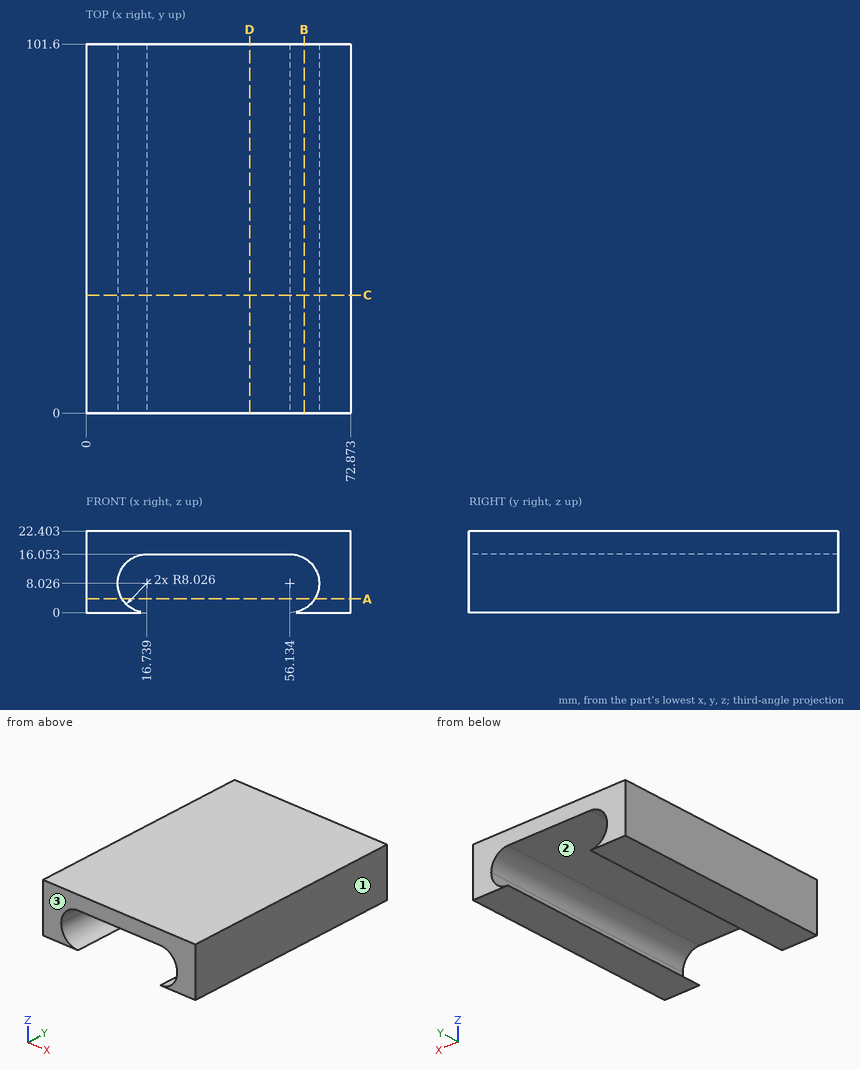
Study the drawing (mm; zero at the part's minimum x, y, z) and answer. Give positions to 0.01 mm unless a question says otherwise; leave off trailing zeros. Order: outer loops, then holes, each group sorted by start corner. A loop starts at its lowest first (then second) coordinate and runs counter-clockwise, first axis right, second up. Notation, with made-up numbers: M 63,86 L 91,86 A9 ccw 91,95 Z; hole C -26.75,62 d11. An arc over 180 degrees is marked long. Put each result on its own line as item: value. Start each with the question number.
Item 1: A flat-ended cylindrical pin translates along its axis: P1, Ø4, axis at x = 13, z = 15.5, coming from the -Y side. Find the tip coordinate at first contact, or state that the pin passes through.
Item 2: The part is cut by section C-C, the plane y = 32.5. Determine the outline of the cut face in (x, z).
Item 3: The part is cut by section B-B, the plane x = 60. Determine the outline of the cut face in (y, z).
Item 4: Find the intervals of material crossed by line 1 along X through (y, z) = (7.5, 7.25); line 2 along Z through (x, y) = (47, 35.5); line 3 along X through (y, z) = (50.5, 4.5) (1 decimal), in increasing order.
Item 5: The part is cut by section D-D, the plane x = 45. Determine the outline of the cut face in (y, z).
Item 6: The part is cut by section A-A, the plane z = 3.75. Determine the outline of the cut face in (x, y), and give its area (3 significant figures).
Item 7: For a pull along X with two mould halves and no side action, classify the marked faces 1, 2 and 3 as +X half, -X half, draft (parallel to the pull), parting line (faces both ways), or undercut.
Answer key:
1. P1: stops at y = 0
2. outline: M 0,0 L 16.74,0 A8.03 cw 8.71,8.03 A8.03 cw 16.74,16.05 L 56.13,16.05 A8.03 cw 64.16,8.03 A8.03 cw 56.13,0 L 72.87,0 L 72.87,22.4 L 0,22.4 Z
3. outline: M 0,0 L 101.6,0 L 101.6,0.99 L 0,0.99 Z; M 0,15.06 L 101.6,15.06 L 101.6,22.4 L 0,22.4 Z
4. line 1: x = 0 to 8.75, 64.12 to 72.87
4. line 2: z = 16.05 to 22.4
4. line 3: x = 0 to 9.5, 63.3 to 72.9
5. outline: M 0,16.05 L 101.6,16.05 L 101.6,22.4 L 0,22.4 Z
6. outline: M 0,0 L 9.95,0 L 9.95,101.6 L 0,101.6 Z; M 62.93,0 L 72.87,0 L 72.87,101.6 L 62.93,101.6 Z
6. area: 2,020 mm²
7. face 1: +X half
7. face 2: undercut
7. face 3: draft
